```python
from build123d import *

# Parameters (mm, degrees)
SKETCH1_W           = 6.9
SKETCH1_H           = 9
BOSS_EXTRUDE1_DEPTH = 1.5
SKETCH2_W           = 1.27616984
SKETCH2_H           = 2
BOSS_EXTRUDE2_DEPTH = 0.3


with BuildPart() as part:
    # Sketch1 → Boss-Extrude1 (new body)
    with BuildSketch(Plane.XY):
        Rectangle(SKETCH1_W, SKETCH1_H)
    extrude(amount=BOSS_EXTRUDE1_DEPTH)

    # Sketch2 → Boss-Extrude2 (add)
    with BuildSketch(Plane.XY):
        Polygon((3.25, 4.5), (3.25, 4.808852059), (2.54, 5.518852059), (-2.54, 5.518852059), (-3.25, 4.808852059), (-3.25, 4.5), align=None)
        with Locations((2.51191508, -5.5)):
            Rectangle(SKETCH2_W, SKETCH2_H)
        with Locations((-2.51191508, -5.5)):
            Rectangle(SKETCH2_W, SKETCH2_H)
    extrude(amount=BOSS_EXTRUDE2_DEPTH)


solid = part.part
```
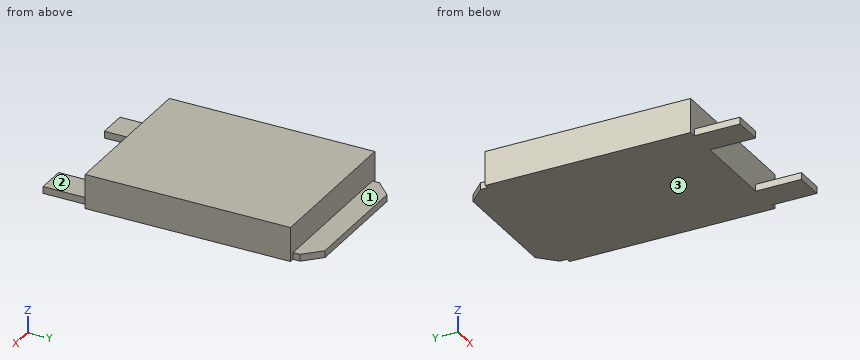
The listing builds one solid part. Answer for the finished solid, in the listing's coordinates (mm). Face numbers are marked on the shaded views. A direction names the side the tool comes from. Round coordinates to 2 decimals unless told otherwise and drop trailing zeros. Write each loop counter-clockwise with the first axis right and the second up, starting at its lowest first coordinate (ties: lowest second). Pieces come first, ordered by that corner, then holes. Notation, with made-up numbers: (-9.5, 32.5) -> (22.5, 32.5) arc R9 ccw to (22.5, 42.5) -> close; hole circle Ø10 at (51.5, -5). An arc over 180 degrees is marked (long way). Answer as a JSON object with one key per item and string values. Group by question number.
Q1. Which of the six approach directions +Z, -Z, +X, -X, +Y, -Y give full straight-line access (tool end or side, diameter ignored) to the marked faces 1, 2 and 3?
Q2. Section C-C (z = 1.15) is taken. Write down the section's boundary in (x, y).
Q3. Section B-B (x = -3) is taken. Write down the section's boundary in (y, z), plus the area to 3 significant figures.
Q4. Section D-D (x = -2) is taken. Write down the section's boundary in (y, z), plus the area to 3 significant figures.
Q5. Each of these flat-tipped pins is pushed along its axis until it touches: pin 1 Ø1.5 at (x, y) = (-1.5, -3) entering from -Z; pin 2 Ø0.8 at (x, y) = (0, 5) entering from +Z. Where does it stop, or does it pass through?
Q6. Section A-A (y = -5.5) is taken. Write down the section's boundary in (x, z).
Q7. Straight lines are drawn through the part: line 1 along Y through (x, z) = (2, 1.35); line 2 along Z through (x, y) = (-2.75, -5.5); line 3 along Y through (x, z) = (1, 0.25). For each, find the intervals that lie inside material, in ascending order.
Check values:
{
 "1": {"face 1": "+Z, +X, -X, +Y", "face 2": "+Z, +X, -X, -Y", "face 3": "-Z, +X, -X, +Y, -Y"},
 "2": {"outline": "(-3.45, -4.5) -> (3.45, -4.5) -> (3.45, 4.5) -> (-3.45, 4.5) -> close"},
 "3": {"outline": "(-6.5, 0) -> (5.06, 0) -> (5.06, 0.3) -> (4.5, 0.3) -> (4.5, 1.5) -> (-4.5, 1.5) -> (-4.5, 0.3) -> (-6.5, 0.3) -> close", "area": "14.3 mm^2"},
 "4": {"outline": "(-6.5, 0) -> (5.52, 0) -> (5.52, 0.3) -> (4.5, 0.3) -> (4.5, 1.5) -> (-4.5, 1.5) -> (-4.5, 0.3) -> (-6.5, 0.3) -> close", "area": "14.4 mm^2"},
 "5": {"pin 1": "z = 0", "pin 2": "z = 0.3"},
 "6": {"outline": "(-3.15, 0) -> (-1.87, 0) -> (-1.87, 0.3) -> (-3.15, 0.3) -> close; (1.87, 0) -> (3.15, 0) -> (3.15, 0.3) -> (1.87, 0.3) -> close"},
 "7": {"line 1": "-4.5 to 4.5", "line 2": "0 to 0.3", "line 3": "-4.5 to 5.52"}
}
